```python
from build123d import *

# Parameters (mm, degrees)
PAD005_DEPTH    = 3
POCKET008_DEPTH = 5
SKETCH040_R     = 1.45
POCKET020_DEPTH = 15
POCKET026_DEPTH = 14
FILLET003_R     = 1.5


with BuildPart() as part:
    # Sketch024 → Pad005 (new body)
    with BuildSketch(Plane.XY):
        with BuildLine():
            Line((85.725, 98.4875), (66.675, 98.4875))
            add(Edge.make_bspline(
                [(-8, 84.2), (39.625, 84.2), (39.625, 98.4875), (66.675, 98.4875)],
                knots=[0, 0, 0, 0, 1, 1, 1, 1], degree=3))
            Line((-8, 84.2), (-8, -8))
            add(Edge.make_bspline(
                [(39.625, -17.525), (39.625, -8), (20.575, -8), (-8, -8)],
                knots=[0, 0, 0, 0, 1, 1, 1, 1], degree=3))
            add(Edge.make_bspline(
                [(153.231854, -38.154949), (107.082107, -17.525), (76.2, -17.525), (39.625, -17.525)],
                knots=[0, 0, 0, 0, 1, 1, 1, 1], degree=3))
            Line((153.231854, -38.154949), (175.310198, 11.234895))
            add(Edge.make_bspline(
                [(150.875, 88.9625), (150.875, 42.8625), (150.875, 22.157965), (175.310198, 11.234895)],
                knots=[0, 0, 0, 0, 1, 1, 1, 1], degree=3))
            add(Edge.make_bspline(
                [(85.725, 98.4875), (104.775, 98.4875), (104.775, 88.9625), (150.875, 88.9625)],
                knots=[0, 0, 0, 0, 1, 1, 1, 1], degree=3))
        make_face()
    extrude(amount=PAD005_DEPTH)

    # Sketch025 → Pocket008 (cut)
    with BuildSketch(Plane(origin=(0, 0, 0), x_dir=(1, 0, 0), z_dir=(0, 0, -1))):
        Polygon((-0.75, 0.75), (-0.75, -76.95), (46.875, -76.95), (46.875, -86.475), (65.925, -86.475), (65.925, -91.2375), (86.475, -91.2375), (86.475, -86.475), (105.525, -86.475), (105.525, -81.7125), (143.625, -81.7125), (143.625, -17.457464), (165.732668, -7.574851), (149.57181, 28.577419), (131.568158, 20.529392), (102.96164, 14.448889), (103.848827, 10.275), (84.975, 10.275), (84.975, 5.5125), (67.425, 5.5125), (67.425, 10.275), (46.875, 10.275), (46.875, 0.75), align=None)
    extrude(amount=-POCKET008_DEPTH, mode=Mode.SUBTRACT)

    # Sketch040 → Pocket020 (cut)
    with BuildSketch(Plane.XY):
        with Locations((-4.375, -4.375)):
            Circle(SKETCH040_R)
        with Locations((-4.375, 80.575)):
            Circle(SKETCH040_R)
        with Locations((151.401832, -33.366184)):
            Circle(SKETCH040_R)
        with Locations((170.521433, 9.404873)):
            Circle(SKETCH040_R)
        with Locations((147.25, 85.3375)):
            Circle(SKETCH040_R)
        with Locations((43.25, -13.9)):
            Circle(SKETCH040_R)
        with Locations((57.15, 92.085)):
            Circle(SKETCH040_R)
        with Locations((95.25, 92.085)):
            Circle(SKETCH040_R)
        with Locations((95.25, -13.9)):
            Circle(SKETCH040_R)
    extrude(amount=POCKET020_DEPTH, mode=Mode.SUBTRACT)

    # Sketch054 → Pocket026 (cut)
    with BuildSketch(Plane.XY):
        Polygon((118.825, 80.9625), (116.825, 92.9625), (166.907578, 98.346489), (154.875, 54.9125), (142.875, 55.9125), align=None)
    extrude(amount=POCKET026_DEPTH, mode=Mode.SUBTRACT)

    # Fillet003
    fillet003_edges = [part.edges().sort_by_distance(p)[0] for p in [
        (-8, -8, 1.5),
        (-8, 84.2, 1.5),
        (175.310198, 11.234895, 1.5),
        (153.231854, -38.154949, 1.5),
        (39.625, -17.525, 1.5),
    ]]
    fillet(fillet003_edges, radius=FILLET003_R)


with BuildPart() as part_1:
    # Body004 placement: moved
    add(part.part.moved(Location((0, 0, -3))))


solid = part_1.part
```
CAD build for the part. Positions are in the model's coordinates, mm. A direction names the side the tool comes from. Give positions to 0.01 mm unless a question says otherwise; leave off trailing zeros. Order: outer loops, then holes, each group sorted by start corner. A loop starts at its lowest first (then second) coordinate and runs counter-clockwise, first axis right, second up. Notation, with made-up numbers: M -35,51 L -13,51 A15 ccw -13,77 Z; hole C 12,-33 d1. An arc over 180 degrees is marked long. Put each result on its own line as item: value. Start each with the question number.
(1) Mould opens along Y. For faces 3 (the flat face through (157.765, -10.248, -1.521)), 4 (the flat face through (154.524, 12.585, -1.521)), 5 (the flat face through (164.13, -13.78, -1.52)), 6 (the flat face through (83, -10, -3)) say: +Y half, -Y half, draft (parallel to the pull), parting line (faces both ways), or undercut.
(2) Which spindle directions (+Z, -Z, +X, -X, +Y, -Y) get a long thin tool onto all of the face, cutting with end or side? Do faces 1 (the flat face through (117.465, -17.532, -1.521)), 2 (the flat face through (83, -10, 0)). Say none if no direction does.
(3) Saw through at B-B, the plane z = -0.85. Give the number of separate pieces and of enclosed holes in the cut face, then the cut area to 3 significant figures.
(4) Drill centre lines: line 1 along Y through (x, z) = (43.25, -1.85); line 2 along X through (y, z) = (49.5, -2.6) (3 decimals); line 3 along Y through (x, z) = (95.25, -2.05) (3 decimals). Where is each one in solid material? Low to high.
(5) Flat gauge pins, fed straight in: pin 1 Ø12 at (x, y) = (18.5, 78) entering from +Z; pin 2 Ø1.5 at (x, z) = (16, -1) entering from -Y; pin 3 Ø2.5 at (x, y) = (-4.375, -4.375) entering from -Z; pin 4 Ø0.9 at (x, z) = (94, -1.5) entering from +Y. Where does each tip first touch, or does it go through?
(6) Saw through at A-A, the plane y = 4. Write the cut outline in (x, z).
Check result:
1. face 3: undercut
1. face 4: undercut
1. face 5: -Y half
1. face 6: draft
2. face 1: +Z, -Z
2. face 2: +Z, +X, -X, +Y, -Y
3. separate pieces: 1
3. enclosed holes: 8
3. area: 4,190 mm2
4. line 1: y = -17.53 to -15.35, -12.45 to -0.75, 76.95 to 93.78
4. line 2: x = -8 to -0.75, 143.625 to 151.895
4. line 3: y = -20.463 to -15.35, -12.45 to -10.275, 86.475 to 90.635, 93.535 to 97.527
5. pin 1: stops at z = 0
5. pin 2: stops at y = -8.34
5. pin 3: passes through
5. pin 4: stops at y = 97.86
6. outline: M -8,-3 L -0.75,-3 L -0.75,0 L -8,0 Z; M 164.13,-3 L 172.08,-3 L 172.08,0 L 164.13,0 Z
